from build123d import *

# Parameters (mm, degrees)
SKETCH_3_R          = 2.45
EXTRUDE_2_DEPTH     = 10
EXTRUDE_2_2_DEPTH   = 10
SKETCH_4_W          = 52
SKETCH_4_H          = 15
EXTRUDE_3_DEPTH     = 5
SKETCH_5_W          = 52
SKETCH_5_H          = 3
CUT_EXTRUDE_1_DEPTH = 31.939457009


with BuildPart() as part:
    # Sketch 3 → Extrude 2 (new body)
    with BuildSketch(Plane.XY):
        with Locations((-21, 0)):
            Circle(SKETCH_3_R)
    extrude(amount=EXTRUDE_2_DEPTH)



with BuildPart() as body_2:
    # Sketch 3 → Extrude 2 2 (new body)
    with BuildSketch(Plane.XY):
        with Locations(Location((21, 0, 0), (0, 0, 180))):
            Circle(SKETCH_3_R)
    extrude(amount=EXTRUDE_2_2_DEPTH)


with BuildPart() as part_1:
    add(part.part)

    add(body_2.part)  # Extrude 3 merges body 2
    # Sketch 4 → Extrude 3 (add)
    with BuildSketch(Plane.XY):
        Rectangle(SKETCH_4_W, SKETCH_4_H)
    extrude(amount=-EXTRUDE_3_DEPTH)

    # Sketch 5 → Cut-Extrude 1 (cut, through all)
    with BuildSketch(Plane(origin=(0, 0, -5), x_dir=(-1, 0, 0), z_dir=(0, 0, -1))):
        with Locations((0, 6)):
            Rectangle(SKETCH_5_W, SKETCH_5_H)
    extrude(amount=-CUT_EXTRUDE_1_DEPTH, mode=Mode.SUBTRACT)


solid = part_1.part
Can you work these out from the model? Positions are in its coordinate system, mm. Coordinates: 2 decimals unless noted, no trailing zeros. Write each loop counter-clockwise with the first axis right and the second up, starting at its lowest first coordinate (ties: lowest second). Pieces come first, ordered by that corner, then holes.
Q1. Imagine slicing it at D-D, the plane x = -13. List the corners of the cut face in (y, z) for me, plus the area to 3 significant figures.
Results found:
outline: (-7.5, -5) - (4.5, -5) - (4.5, 0) - (-7.5, 0) - close
area: 60.0 mm2
Q2. Please list where these lines run through material, in increasing order: L1, parallel to Z at x = -1.5, y = -4.5; L2, parallel to Y at x = -20.5, z = 1.75; L3, parallel to Y at x = -22, z = 0.25.
Results found:
L1: z = -5 to 0
L2: y = -2.4 to 2.4
L3: y = -2.24 to 2.24
Q3. For P1, Ø5, axis at x = -3, y = -0.5, coming from the +Z side; P2, Ø6, axis at y = -5, z = 7, coming from the +X side; P3, Ø4, axis at y = -1, z = 6, coming from the +X side, each with a flat end and sliding along its axis, tell me the tip position at first contact or that it passes through.
Results found:
P1: stops at z = 0
P2: stops at x = 22.42
P3: stops at x = 23.45
Q4. Imagine slicing it at C-C, the plane y = 0. List the corners of the cut face in (x, z) for me.
Results found:
outline: (-26, -5) - (26, -5) - (26, 0) - (23.45, 0) - (23.45, 10) - (18.55, 10) - (18.55, 0) - (-18.55, 0) - (-18.55, 10) - (-23.45, 10) - (-23.45, 0) - (-26, 0) - close
Q5. Imagine slicing it at B-B, the plane x = -21. List the corners of the cut face in (y, z) for me.
Results found:
outline: (-7.5, -5) - (4.5, -5) - (4.5, 0) - (2.45, 0) - (2.45, 10) - (-2.45, 10) - (-2.45, 0) - (-7.5, 0) - close
Q6. Imagine slicing it at A-A, the plane z = 3.25. List the corners of the cut face in (x, y) for me.
Results found:
outline: circle Ø4.9 at (-21, 0); circle Ø4.9 at (21, 0)
Q7. If we mould it in two halves opening along X, with no side actions, what happens to faces 1 (the face through (0, -1, -5)), 2 (the face through (-23.448, 0.108, 4.93)), 3 (the face through (23.448, -0.108, 4.93)), 4 (the face through (26, -2, -2))? For each: +X half, -X half, draft (parallel to the pull), parting line (faces both ways), or undercut.
Results found:
face 1: draft
face 2: undercut
face 3: undercut
face 4: +X half
